Here's how the part is built. I have some questions about the finished solid (model axes, mm). A direction names the side the tool comes from. Coordinates: 2 decimals unless noted, no trailing zeros. Write each loop counter-clockwise with the first axis right and the second up, starting at its lowest first coordinate (ties: lowest second). Pieces come first, ordered by that corner, then holes.
(1) Imagine slicing it at A-A, the plane z = 0. List the corners of the cut face in (x, y) for me.
(2) Which directions (+Z, -Z, +X, -X, +Y, -Y) give clear straight access to the entire face, cutting with the end or side of a thin tool? Please do faces 1 (the flat face through (-4.5, 0.5, -7.4)), 2 (the flat face through (-3, 0, -10)), 3 (the cylindrical face through (4.57, 3.754, -7.167)).
(3) Please list where these lines run through material, in increasing order: probe 1 along Z at (x, y) = (0, 2.5); probe 2 along X at (y, z) = (3.8, 1.75); probe 3 along Y at (x, z) = (-0.75, 8.5).
(4) For pin 1 Ø1.5 at (x, y) = (-5.5, 2) entering from -Z, with a flat end and sliding along its axis, tell me the tip position at first contact or that it passes through.
(5) Thinking about a two-plate mould opening in Z: for faces 4 (the flat face through (-3, 4, -10)), 5 (the cylindrical face through (2.38, 1.98, 10.74)), 6 (the cylindrical face through (4.57, 0.246, 7.167)), which applies, released by +Z, released by -Z, zero draft, split by the parting line, or undercut?
(6) Imagine slicing it at C-C, the plane y = 1.85. List the corners of the cut face in (x, z) for me.
(7) Imagine slicing it at B-B, the plane x = 0. List the corners of the cut face in (y, z) for me, plus the area to 3 significant figures.
Autodesk Inventor part; units mm, degrees
ref_plane "YZ Plane" through (0, 0, 0) normal (1, 0, 0) x (0, 1, 0)
ref_plane "XZ Plane" through (0, 0, 0) normal (0, 1, 0) x (-1, 0, 0)
ref_plane "XY Plane" through (0, 0, 0) normal (0, 0, 1) x (1, 0, 0)
sketch "Sketch1" plane through (0, 0, 0) normal (0, 1, 0) x (-1, 0, 0)
  circle A0 centre (0, 0) radius 8
  circle A1 centre (0, 0) radius 11
  dimension "d0" = 16
  dimension "d1" = 22
extrude "Extrusion1" add sketch "Sketch1" along normal blind 4
chamfer "Chamfer1" distance 0.25 angle 45 2 edges at (11, 4, 0) (11, 0, 0)
sketch "Sketch2" plane through (0, 4, 0) normal (0, 1, 0) x (1, 0, 0)
  circle A0 centre (0, 0) radius 8 construction
  circle A1 centre (0, 0) radius 8.5
  circle A2 centre (0, 0) radius 10
  dimension "d7" = 0.5
  dimension "d8" = 1.5
extrude "Extrusion2" cut sketch "Sketch2" against normal blind 0.5
sketch "Sketch3" plane through (0, 0, 0) normal (0, -1, 0) x (1, 0, 0)
  circle A0 centre (0, 0) radius 10
  circle A1 centre (0, 0) radius 8.5
extrude "Extrusion3" cut sketch "Sketch3" against normal blind 0.5
properties part number "16mm ID x 22mm OD x 4mm Thickness Ball Bearing"
Recorded:
1. outline: (-11, 0.25) - (-10.75, 0) - (-10, 0) - (-10, 0.5) - (-8.5, 0.5) - (-8.5, 0) - (-8, 0) - (-8, 4) - (-8.5, 4) - (-8.5, 3.5) - (-10, 3.5) - (-10, 4) - (-10.75, 4) - (-11, 3.75) - close; (8, 0) - (8.5, 0) - (8.5, 0.5) - (10, 0.5) - (10, 0) - (10.75, 0) - (11, 0.25) - (11, 3.75) - (10.75, 4) - (10, 4) - (10, 3.5) - (8.5, 3.5) - (8.5, 4) - (8, 4) - close
2. face 1: -Y
2. face 2: +Z, -Z, +X, -X, -Y
2. face 3: +Y
3. probe 1: z = -11 to -8, 8 to 11
3. probe 2: x = -10.81 to -9.85, -8.32 to -7.81, 7.81 to 8.32, 9.85 to 10.81
3. probe 3: y = 0.5 to 3.5
4. pin 1: stops at z = -9.92
5. face 4: zero draft
5. face 5: split by the parting line
5. face 6: undercut
6. outline: circle Ø22 at (0, 0); hole circle Ø16 at (0, 0)
7. outline: (0, -10.75) - (0.25, -11) - (3.75, -11) - (4, -10.75) - (4, -10) - (3.5, -10) - (3.5, -8.5) - (4, -8.5) - (4, -8) - (0, -8) - (0, -8.5) - (0.5, -8.5) - (0.5, -10) - (0, -10) - close; (0, 8) - (4, 8) - (4, 8.5) - (3.5, 8.5) - (3.5, 10) - (4, 10) - (4, 10.75) - (3.75, 11) - (0.25, 11) - (0, 10.75) - (0, 10) - (0.5, 10) - (0.5, 8.5) - (0, 8.5) - close
7. area: 20.9 mm2
